from build123d import *

# Parameters (mm, degrees)
F1_R     = 3.175
F1_R_2   = 5
F2_DEPTH = 25
F3_R     = 25.4


with BuildPart() as f2:
    # F1 (on Top) → F2 (new body)
    with BuildSketch(Plane.XY):
        with BuildLine():
            ThreePointArc((-71.110451, 54.240226), (-77.927858, 45.597173), (-87.921111, 50.213914))
            ThreePointArc((-87.921111, 50.213914), (-42.888123, 0.321655), (21.151845, -20.076632))
            Line((21.151845, -20.076632), (37.572558, -20.804112))
            ThreePointArc((37.572558, -20.804112), (50.822204, -8.678648), (38.69674, 4.570998))
            Line((38.69674, 4.570998), (21.151845, 5.348282))
            ThreePointArc((21.151845, 5.348282), (-14.99621, 16.862317), (-40.41557, 45.024544))
            Line((-40.41557, 45.024544), (-52.261319, 68.33515))
            ThreePointArc((-52.261319, 68.33515), (-51.541425, 66.37893), (-51.296978, 64.308837))
            ThreePointArc((-51.296978, 64.308837), (-68.207732, 60.485871), (-54.585882, 71.211255))
            Line((-54.585882, 71.211255), (-73.106711, 86.233619))
            Line((-73.106711, 86.233619), (-84.613695, 108.877588))
            Line((-84.613695, 108.877588), (-85.829489, 132.69385))
            ThreePointArc((-85.829489, 132.69385), (-85.820821, 132.46737), (-85.817931, 132.240743))
            ThreePointArc((-85.817931, 132.240743), (-99.353216, 124.665405), (-98.731743, 140.163903))
            Line((-98.731743, 140.163903), (-118.545215, 130.095292))
            ThreePointArc((-118.545215, 130.095292), (-109.871118, 129.74747), (-105.631403, 122.172132))
            ThreePointArc((-105.631403, 122.172132), (-110.695938, 114.148879), (-120.117499, 115.269714))
            Line((-120.117499, 115.269714), (-101.596671, 100.24735))
            Line((-101.596671, 100.24735), (-90.089687, 77.603381))
            Line((-90.089687, 77.603381), (-88.873893, 53.787119))
            ThreePointArc((-88.873893, 53.787119), (-80.224578, 63.124836), (-71.110451, 54.240226))
        make_face()
        with Locations((21.151845, -7.364175)):
            Circle(F1_R, mode=Mode.SUBTRACT)
        with Locations((38.134649, -8.116557)):
            Circle(F1_R, mode=Mode.SUBTRACT)
        with BuildLine():
            ThreePointArc((-118.545215, 130.095292), (-122.968456, 124.92762), (-122.442064, 118.14582))
            ThreePointArc((-122.442064, 118.14582), (-121.431028, 116.585524), (-120.117499, 115.269714))
            ThreePointArc((-120.117499, 115.269714), (-110.695938, 114.148879), (-105.631403, 122.172132))
            ThreePointArc((-105.631403, 122.172132), (-109.871118, 129.74747), (-118.545215, 130.095292))
        make_face()
        with Locations((-114.518903, 122.172132)):
            Circle(F1_R_2, mode=Mode.SUBTRACT)
        with BuildLine():
            ThreePointArc((-86.78227, 136.267055), (-91.949943, 140.690296), (-98.731743, 140.163903))
            ThreePointArc((-98.731743, 140.163903), (-99.353216, 124.665405), (-85.817931, 132.240743))
            ThreePointArc((-85.817931, 132.240743), (-85.820821, 132.46737), (-85.829489, 132.69385))
            ThreePointArc((-85.829489, 132.69385), (-86.117974, 134.530557), (-86.78227, 136.267055))
        make_face()
        with Locations((-94.705431, 132.240743)):
            Circle(F1_R_2, mode=Mode.SUBTRACT)
        with BuildLine():
            ThreePointArc((-88.873893, 53.787119), (-88.585408, 51.950412), (-87.921111, 50.213914))
            ThreePointArc((-87.921111, 50.213914), (-77.927858, 45.597173), (-71.110451, 54.240226))
            ThreePointArc((-71.110451, 54.240226), (-80.224578, 63.124836), (-88.873893, 53.787119))
        make_face()
        with Locations((-79.997951, 54.240226)):
            Circle(F1_R_2, mode=Mode.SUBTRACT)
        with BuildLine():
            ThreePointArc((-51.296978, 64.308837), (-51.541425, 66.37893), (-52.261319, 68.33515))
            ThreePointArc((-52.261319, 68.33515), (-53.272354, 69.895445), (-54.585882, 71.211255))
            ThreePointArc((-54.585882, 71.211255), (-68.207732, 60.485871), (-51.296978, 64.308837))
        make_face()
        with Locations((-60.184478, 64.308837)):
            Circle(F1_R_2, mode=Mode.SUBTRACT)
    extrude(amount=F2_DEPTH)

    # F3
    f3_edges = [f2.edges().sort_by_distance(p)[0] for p in [
        (-73.106711, 86.233619, 12.5),
        (-84.613695, 108.877588, 12.5),
        (-101.596671, 100.24735, 12.5),
        (-90.089687, 77.603381, 12.5),
    ]]
    fillet(f3_edges, radius=F3_R)


solid = f2.part
Here's how the part is built. I have some questions about the finished solid (model axes, mm). Round coordinates to 2 decimals unless told otherwise and drop trailing zeros. Loops run counter-clockwise (first coordinate to the right, second up) from the corner with the lowest first, then second, coordinate; pieces in that order, holes last. Notation, with made-up numbers: (52, -19) - (102, -19) arc R14 ccw to (102, -10) - close; hole circle Ø9 at (-10.75, 68). An arc over 180 degrees is marked (long way). One line per question, with ' | ' between items. Start each with the question number.
Q1. I want a section at C-C (y = -0.5). Write out the boundary of the cut face in (x, z).
Q2. I want a section at B-B (z = 18.75). State how many separate pieces and enclosed holes the cut face has, then the cut area to 3 significant figures.
Q3. I want a section at A-A (x = -79.5). Write out the boundary of the cut face in (y, z), then the cut area to 3 significant figures.
Q4. I want a section at D-D (x = -22). Write out the boundary of the cut face in (y, z).
Q5. We'd pull the mould along X, two halves only. Please class faces 1 (the cylindrical face through (-91.86, 140.66, 12.32)), 2 (the cylindrical face through (24.085, -8.58, 12.325)), 3 (the cylindrical face through (-90.62, 77.38, 12.68)), 4 (the cylindrical face through (34.963, -7.977, 12.325)): +X half, -X half, draft (parallel to the pull), parting line (faces both ways), or undercut.
Q6. Please list where these lines run through material, in increasing order: line 1 (Y direction, x = -56, z = 18); line 2 (X direction, y = 54, z = 17.5); line 3 (Y direction, x = -114.5, z = 8.5). Write a range as [from, to].
Q7. Will these pins go through, and if not, where does the flat tip stop? pin 1 (1.5 mm diameter, centred on y = 23.5, z = 17.5, fed in from -X); pin 2 (5 mm diameter, centred on x = 5, z = 20.5, fed in from +Y); pin 3 (4 mm diameter, centred on x = 38.13, y = -8.12, fed in from -Z); pin 4 (1.5 mm diameter, centred on y = 67.5, z = 9.5, fed in from -X).
Response values:
1) outline: (-41.6, 0) - (48.3, 0) - (48.3, 25) - (-41.6, 25) - close
2) separate pieces: 1 | enclosed holes: 6 | area: 6,400 mm²
3) outline: (35.99, 0) - (49.27, 0) - (49.27, 25) - (35.99, 25) - close; (59.22, 0) - (98.81, 0) - (98.81, 25) - (59.22, 25) - close | area: 1,320 mm²
4) outline: (-10.57, 0) - (21.99, 0) - (21.99, 25) - (-10.57, 25) - close
5) face 1: parting line | face 2: undercut | face 3: -X half | face 4: undercut
6) line 1: y = [10, 61.57], [67.05, 72.36] | line 2: x = [-88.88, -84.99], [-75, -44.98] | line 3: y = [110.71, 117.17], [127.17, 132.15]
7) pin 1: stops at x = -70.46 | pin 2: stops at y = 8.65 | pin 3: passes through | pin 4: stops at x = -89.61
